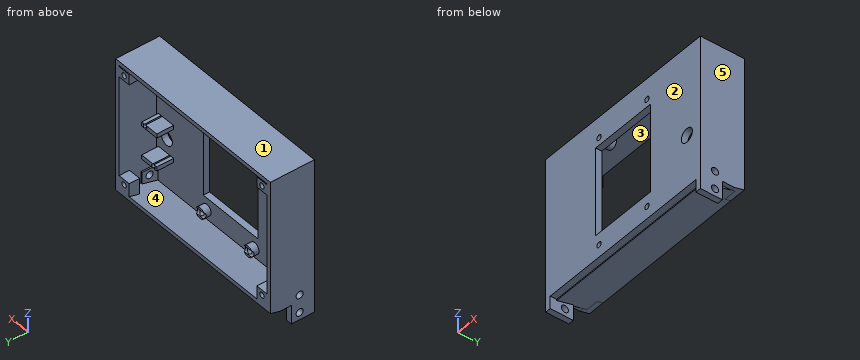
from build123d import *

# Parameters (mm, degrees)
SKETCH_1_W                                 = 92
SKETCH_1_H                                 = 3
FRONT_PANEL_1_DEPTH                        = 65
SKETCH_2_W                                 = 32.6
SKETCH_2_H                                 = 42.6
STEP_PORTRAIT_LCD_WINDOW_32_6X42_6_2_DEPTH = 5
SKETCH_3_R                                 = 3.3
BUTTON_BORE_3_DEPTH                        = 5
SKETCH_4_R                                 = 2.6
FOUR_M3_PCB_STANDOFFS_4_DEPTH              = 3.2
SKETCH_5_R                                 = 1.3
M3_PCB_MOUNT_PILOTS_52X28_5_5_DEPTH        = 9
SKETCH_6_W                                 = 2
SKETCH_6_H                                 = 18
HOUSING_LEFT_6_DEPTH                       = 65
SKETCH_7_W                                 = 2
SKETCH_7_H                                 = 18
HOUSING_RIGHT_7_DEPTH                      = 65
SKETCH_9_W                                 = 88
SKETCH_9_H                                 = 18
HOUSING_TOP_9_DEPTH                        = 2
SKETCH_10_W                                = 6
SKETCH_10_H                                = 5
COVER_POST_LB_10_DEPTH                     = 5
SKETCH_11_W                                = 6
SKETCH_11_H                                = 5
COVER_POST_RB_11_DEPTH                     = 5
SKETCH_12_W                                = 6
SKETCH_12_H                                = 5
COVER_POST_LT_12_DEPTH                     = 5
SKETCH_13_W                                = 6
SKETCH_13_H                                = 5
COVER_POST_RT_13_DEPTH                     = 5
SKETCH_15_W                                = 9
SKETCH_15_H                                = 8
BUTTON_LOWER_SHELF_15_DEPTH                = 2
SKETCH_16_W                                = 9
SKETCH_16_H                                = 8
BUTTON_UPPER_SHELF_16_DEPTH                = 2
SKETCH_17_R                                = 1.05
BUTTON_CARRIER_M2_PILOTS_17_DEPTH          = 10
SKETCH_18_W                                = 2.7
SKETCH_18_H                                = 10.5
RIGHT_TILT_EAR_18_DEPTH                    = 15
SKETCH_19_W                                = 2.7
SKETCH_19_H                                = 11
LEFT_TILT_EAR_19_DEPTH                     = 15
SKETCH_20_R                                = 1.7
M3_HINGE_AND_ANGLE_LOCK_20_DEPTH           = 94
SKETCH_21_W                                = 92
SKETCH_21_H                                = 3
FRONT_LOWER_EXTENSION_201_DEPTH            = 3
HOUSING_CAGE_ROOF_CLEARANCE_202_DEPTH      = 94
HORIZONTAL_ENCLOSURE_FLOOR_203_DEPTH       = 88
SKETCH_24_W                                = 6
SKETCH_24_H                                = 5
COVER_LOWER_POST_L_204_DEPTH               = 5
SKETCH_25_W                                = 6
SKETCH_25_H                                = 5
COVER_LOWER_POST_R_205_DEPTH               = 5
SKETCH_26_R                                = 1.3
REAR_COVER_M3_PILOTS_FINAL_206_DEPTH       = 8


with BuildPart() as part:
    # Эскиз1 → Front_panel_1 (new body)
    with BuildSketch(Plane.XY.offset(55)):
        with Locations((0, -65.5)):
            Rectangle(SKETCH_1_W, SKETCH_1_H)
    extrude(amount=FRONT_PANEL_1_DEPTH)

    # Эскиз2 → STEP_portrait_LCD_window_32_6x42_6_2 (cut)
    with BuildSketch(Plane(origin=(0, -68, 0), x_dir=(1, 0, 0), z_dir=(0, 1, 0))):
        with Locations((0, -85)):
            Rectangle(SKETCH_2_W, SKETCH_2_H)
    extrude(amount=STEP_PORTRAIT_LCD_WINDOW_32_6X42_6_2_DEPTH, mode=Mode.SUBTRACT)

    # Эскиз3 → Button_bore_3 (cut)
    with BuildSketch(Plane(origin=(0, -68, 0), x_dir=(1, 0, 0), z_dir=(0, 1, 0))):
        with Locations(Location((38, -77, 0), (0, 0, 90))):
            Circle(SKETCH_3_R)
    extrude(amount=BUTTON_BORE_3_DEPTH, mode=Mode.SUBTRACT)

    # Эскиз4 → Four_M3_PCB_standoffs_4 (add)
    with BuildSketch(Plane(origin=(0, -64, 0), x_dir=(1, 0, 0), z_dir=(0, 1, 0))):
        with Locations(Location((-14.25, -58, 0), (0, 0, 90))):
            Circle(SKETCH_4_R)
        with Locations(Location((-14.25, -110, 0), (0, 0, 90))):
            Circle(SKETCH_4_R)
        with Locations(Location((14.25, -58, 0), (0, 0, 90))):
            Circle(SKETCH_4_R)
        with Locations(Location((14.25, -110, 0), (0, 0, 90))):
            Circle(SKETCH_4_R)
    extrude(amount=FOUR_M3_PCB_STANDOFFS_4_DEPTH)

    # Эскиз5 → M3_PCB_mount_pilots_52x28_5_5 (cut)
    with BuildSketch(Plane(origin=(0, -68, 0), x_dir=(1, 0, 0), z_dir=(0, 1, 0))):
        with Locations(Location((-14.25, -58, 0), (0, 0, 270))):
            Circle(SKETCH_5_R)
        with Locations(Location((14.25, -58, 0), (0, 0, 270))):
            Circle(SKETCH_5_R)
        with Locations(Location((-14.25, -110, 0), (0, 0, 270))):
            Circle(SKETCH_5_R)
        with Locations(Location((14.25, -110, 0), (0, 0, 270))):
            Circle(SKETCH_5_R)
    extrude(amount=M3_PCB_MOUNT_PILOTS_52X28_5_5_DEPTH, mode=Mode.SUBTRACT)

    # Эскиз6 → Housing_left_6 (add)
    with BuildSketch(Plane.XY.offset(55)):
        with Locations((-45, -55)):
            Rectangle(SKETCH_6_W, SKETCH_6_H)
    extrude(amount=HOUSING_LEFT_6_DEPTH)

    # Эскиз7 → Housing_right_7 (add)
    with BuildSketch(Plane.XY.offset(55)):
        with Locations((45, -55)):
            Rectangle(SKETCH_7_W, SKETCH_7_H)
    extrude(amount=HOUSING_RIGHT_7_DEPTH)

    # Эскиз9 → Housing_top_9 (add)
    with BuildSketch(Plane.XY.offset(118)):
        with Locations((0, -55)):
            Rectangle(SKETCH_9_W, SKETCH_9_H)
    extrude(amount=HOUSING_TOP_9_DEPTH)

    # Эскиз10 → Cover_post_LB_10 (add)
    with BuildSketch(Plane.XY.offset(55.5)):
        with Locations((-41, -48.5)):
            Rectangle(SKETCH_10_W, SKETCH_10_H)
    extrude(amount=COVER_POST_LB_10_DEPTH)

    # Эскиз11 → Cover_post_RB_11 (add)
    with BuildSketch(Plane.XY.offset(55.5)):
        with Locations((41, -48.5)):
            Rectangle(SKETCH_11_W, SKETCH_11_H)
    extrude(amount=COVER_POST_RB_11_DEPTH)

    # Эскиз12 → Cover_post_LT_12 (add)
    with BuildSketch(Plane.XY.offset(112.5)):
        with Locations((-41, -48.5)):
            Rectangle(SKETCH_12_W, SKETCH_12_H)
    extrude(amount=COVER_POST_LT_12_DEPTH)

    # Эскиз13 → Cover_post_RT_13 (add)
    with BuildSketch(Plane.XY.offset(112.5)):
        with Locations((41, -48.5)):
            Rectangle(SKETCH_13_W, SKETCH_13_H)
    extrude(amount=COVER_POST_RT_13_DEPTH)

    # Эскиз15 → Button_lower_shelf_15 (add)
    with BuildSketch(Plane.XY.offset(68)):
        with Locations((38.5, -60)):
            Rectangle(SKETCH_15_W, SKETCH_15_H)
    extrude(amount=BUTTON_LOWER_SHELF_15_DEPTH)

    # Эскиз16 → Button_upper_shelf_16 (add)
    with BuildSketch(Plane.XY.offset(84)):
        with Locations((38.5, -60)):
            Rectangle(SKETCH_16_W, SKETCH_16_H)
    extrude(amount=BUTTON_UPPER_SHELF_16_DEPTH)

    # Эскиз17 → Button_carrier_M2_pilots_17 (cut)
    with BuildSketch(Plane(origin=(0, -65, 0), x_dir=(1, 0, 0), z_dir=(0, 1, 0))):
        with Locations(Location((36, -69, 0), (0, 0, 72.247209838))):
            Circle(SKETCH_17_R)
        with Locations(Location((41, -85, 0), (0, 0, 72.247209838))):
            Circle(SKETCH_17_R)
    extrude(amount=BUTTON_CARRIER_M2_PILOTS_17_DEPTH, mode=Mode.SUBTRACT)

    # Эскиз18 → Right_tilt_ear_18 (add)
    with BuildSketch(Plane.XY.offset(46)):
        with Locations((44.65, -61.75)):
            Rectangle(SKETCH_18_W, SKETCH_18_H)
    extrude(amount=RIGHT_TILT_EAR_18_DEPTH)

    # Эскиз19 → Left_tilt_ear_19 (add)
    with BuildSketch(Plane.XY.offset(46)):
        with Locations((-44.65, -61.5)):
            Rectangle(SKETCH_19_W, SKETCH_19_H)
    extrude(amount=LEFT_TILT_EAR_19_DEPTH)

    # Эскиз20 → M3_hinge_and_angle_lock_20 (cut)
    with BuildSketch(Plane(origin=(-47, 0, 0), x_dir=(0, 0, -1), z_dir=(1, 0, 0))):
        with Locations(Location((-49.5, -60, 0), (0, 0, 180))):
            Circle(SKETCH_20_R)
        with Locations(Location((-58, -60, 0), (0, 0, 180))):
            Circle(SKETCH_20_R)
    extrude(amount=M3_HINGE_AND_ANGLE_LOCK_20_DEPTH, mode=Mode.SUBTRACT)

    # Эскиз21 → Front_lower_extension_201 (add)
    with BuildSketch(Plane.XY.offset(52)):
        with Locations((0, -65.5)):
            Rectangle(SKETCH_21_W, SKETCH_21_H)
    extrude(amount=FRONT_LOWER_EXTENSION_201_DEPTH)

    # Эскиз22 → Housing_cage_roof_clearance_202 (cut)
    with BuildSketch(Plane(origin=(-47, 0, 0), x_dir=(0, 0, -1), z_dir=(1, 0, 0))):
        Polygon((-10, -55), (-10, -40), (-57.861284772, -40), (-53.842046885, -55), align=None)
    extrude(amount=HOUSING_CAGE_ROOF_CLEARANCE_202_DEPTH, mode=Mode.SUBTRACT)

    # Эскиз23 → Horizontal_enclosure_floor_203 (add)
    with BuildSketch(Plane(origin=(-44, 0, 0), x_dir=(0, 0, -1), z_dir=(1, 0, 0))):
        Polygon((-51.430504153, -64), (-56.253589617, -46), (-58.22061436, -46), (-53.397528896, -64), align=None)
    extrude(amount=HORIZONTAL_ENCLOSURE_FLOOR_203_DEPTH)

    # Эскиз24 → Cover_lower_post_L_204 (add)
    with BuildSketch(Plane.XY.offset(59.5)):
        with Locations((-41, -48.5)):
            Rectangle(SKETCH_24_W, SKETCH_24_H)
    extrude(amount=COVER_LOWER_POST_L_204_DEPTH)

    # Эскиз25 → Cover_lower_post_R_205 (add)
    with BuildSketch(Plane.XY.offset(59.5)):
        with Locations((41, -48.5)):
            Rectangle(SKETCH_25_W, SKETCH_25_H)
    extrude(amount=COVER_LOWER_POST_R_205_DEPTH)

    # Эскиз26 → Rear_cover_M3_pilots_final_206 (cut)
    with BuildSketch(Plane(origin=(0, -52, 0), x_dir=(1, 0, 0), z_dir=(0, 1, 0))):
        with Locations(Location((-41, -62, 0), (0, 0, 90))):
            Circle(SKETCH_26_R)
        with Locations(Location((41, -62, 0), (0, 0, 90))):
            Circle(SKETCH_26_R)
        with Locations(Location((-41, -115, 0), (0, 0, 90))):
            Circle(SKETCH_26_R)
        with Locations(Location((41, -115, 0), (0, 0, 90))):
            Circle(SKETCH_26_R)
    extrude(amount=REAR_COVER_M3_PILOTS_FINAL_206_DEPTH, mode=Mode.SUBTRACT)


solid = part.part
Can you work these out from the model? Positions are in its coordinate system, mm. Face numbers are marked on the shaded views. A direction names the side the tool comes from. Round coordinates to 2 decimals unless told otherwise and drop trailing zeros. Write each loop counter-clockwise with the first axis right and the second up, starting at its lowest first coordinate (ties: lowest second). Pieces come first, ordered by that corner, then holes. Notation, with made-up numbers: (46, 44.25) -> (56, 44.25) arc R24 cw to (56, 77.25) -> close; hole circle Ø2 at (-17.75, 6.5). An arc over 180 degrees is marked (long way). Use one line per item in the form item = value. Start each with the question number.
Q1. We'd pull the mould along Z, two halves only. Please class the marked faces 1, 2 and 3: +Z half, -Z half, draft (parallel to the pull), parting line (faces both ways), or undercut.
Q2. Imagine slicing it at A-A (z = 49.5). Please give me the cut outline in (x, y), then the cut area to 3 significant figures.
Q3. Imagine slicing it at C-C (z = 95.5). Please give me the cut outline in (x, y).
Q4. Which directions (+Z, -Z, +X, -X, +Y, -Y) give clear straight access to the entire face, cutting with the end or side of a thin tool? Please do the marked faces 4 and 5.
Q5. I'm going to push flat-ended pins straight in: P1, Ø1, axis at x = 40.5, z = 85.5, coming from the +Y side; P2, Ø3.5, axis at x = 9.5, y = -66, coming from the -Z side; P3, Ø2, axis at x = -34, z = 66.5, coming from the +Y side. Where does each tip first touch, or does it pass through?
Q6. If I drill on probe 1 along X at (y, z) = (-64.5, 110); probe 2 along X at (y, z) = (-62, 110); probe 3 along X at (y, z) = (-50, 74.5), over which ranges is the centre line in solid material (lowest first)? Write a range as [from, to].
Q7. Imagine slicing it at B-B (x = -14.25). Count the separate pieces of the cut face and the enclosed holes in it, then the cut area to 3 significant figures.
Q8. Imagine slicing it at D-D (z = 115). Please give me the cut outline in (x, y), then the cut area to 3 significant figures.
Worked out:
q1.face_1 = +Z half
q1.face_2 = draft
q1.face_3 = undercut
q2.outline = (-46, -67) -> (-43.3, -67) -> (-43.3, -61.7) -> (-46, -61.7) -> close; (-46, -58.3) -> (-43.3, -58.3) -> (-43.3, -56) -> (-46, -56) -> close; (43.3, -67) -> (46, -67) -> (46, -61.7) -> (43.3, -61.7) -> close; (43.3, -58.3) -> (46, -58.3) -> (46, -56.5) -> (43.3, -56.5) -> close
q2.area = 39.7 mm^2
q3.outline = (-46, -67) -> (-16.3, -67) -> (-16.3, -64) -> (-44, -64) -> (-44, -46) -> (-46, -46) -> close; (16.3, -67) -> (46, -67) -> (46, -46) -> (44, -46) -> (44, -64) -> (16.3, -64) -> close
q4.face_4 = none
q4.face_5 = +Z, -Z, +X, +Y, -Y
q5.P1 = -56
q5.P2 = 52
q5.P3 = -64
q6.probe_1 = [-46, -15.55], [-12.95, 12.95], [15.55, 46]
q6.probe_2 = [-46, -44], [-16.85, -15.55], [-12.95, -11.65], [11.65, 12.95], [15.55, 16.85], [44, 46]
q6.probe_3 = [-46, -44], [44, 46]
q7.separate_pieces = 4
q7.enclosed_holes = 0
q7.area = 149 mm^2
q8.outline = (-46, -67) -> (46, -67) -> (46, -46) -> (42.3, -46) -> (42.3, -51) -> (44, -51) -> (44, -64) -> (-44, -64) -> (-44, -51) -> (-42.3, -51) -> (-42.3, -46) -> (-46, -46) -> close; (-39.7, -51) -> (-38, -51) -> (-38, -46) -> (-39.7, -46) -> close; (38, -51) -> (39.7, -51) -> (39.7, -46) -> (38, -46) -> close
q8.area = 382 mm^2
